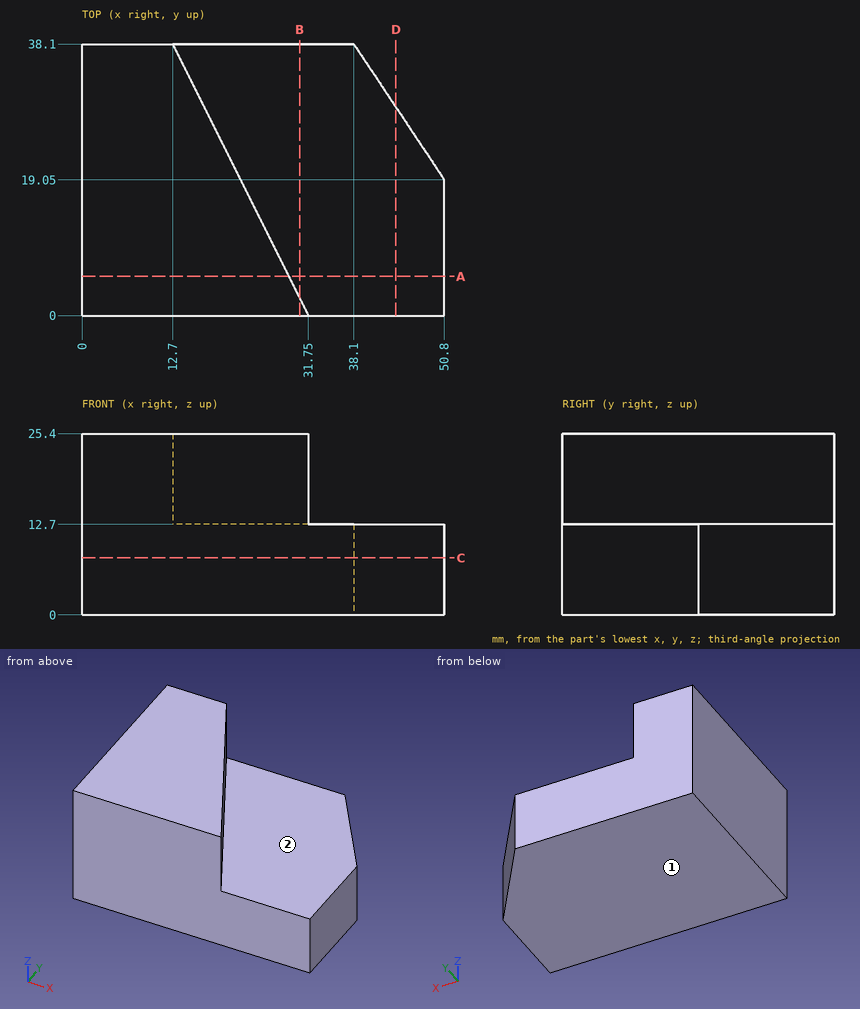
Input: dimensioned drawing with shaded views. Units: mm. Origin: part minimum x, y, z. A direction names the side the tool comes from. Round coordinates to 2 decimals unless told otherwise and drop trailing zeros. Order: outer loops, then holes, each group sorted by start corner. A loop starts at its lowest first (then second) coordinate and runs counter-clockwise, first axis right, second up. Notation, with made-up numbers: (-3, -34.75) - (48, -34.75) arc R4 cw to (48, -27.75) - close; hole circle Ø10 at (-32, -35). An arc over 180 degrees is marked (long way). Answer as a JSON object with one key per item and string values. Group by question number.
(1) Cut plane C-C (z = 8). Return loops of the section in (x, y).
(2) Cut plane B-B (x = 30.5). Return loops of the section in (y, z).
(3) Material intervals for probe 1 along Z at (x, y) = (30, 11); probe 2 along Y at (x, z) = (29.5, 16.25); probe 3 along X at (y, z) = (20, 20.5), sorted ascending. Write a range as from..to.
(4) Cut plane A-A (y = 5.5). Return loops of the section in (x, z).
(5) Pin query (flat end, axial travel): P1, Ø2, axis at x = 20.5, y = 28, coming from the +Z side; P2, Ø10, axis at y = 24.5, z = 13.5, coming from the +X side; P3, Ø12, axis at y = 32, z = 4.5, coming from the +X side. Return the tip coordinate at first contact, or that it passes through.
(6) Reachability of the marked faces 1 and 2 from +Z, -Z, +X, -X, +Y, -Y: full face, straight path, thin tool, end or side. Return the list, or none.
(7) Cut plane D-D (x = 44). Return loops of the section in (y, z), then the cut area to 3 significant figures.
Here are the results:
{
 "1": {"outline": "(0, 0) - (50.8, 0) - (50.8, 19.05) - (38.1, 38.1) - (0, 38.1) - close"},
 "2": {"outline": "(0, 0) - (38.1, 0) - (38.1, 12.7) - (2.5, 12.7) - (2.5, 25.4) - (0, 25.4) - close"},
 "3": {"probe 1": "z = 0..12.7", "probe 2": "y = 0..4.5", "probe 3": "x = 0..21.75"},
 "4": {"outline": "(0, 0) - (50.8, 0) - (50.8, 12.7) - (29, 12.7) - (29, 25.4) - (0, 25.4) - close"},
 "5": {"P1": "stops at z = 12.7", "P2": "stops at x = 50.46", "P3": "stops at x = 46.17"},
 "6": {"face 1": "-Z, +X, -X, +Y, -Y", "face 2": "+Z, +X, +Y"},
 "7": {"outline": "(0, 0) - (29.25, 0) - (29.25, 12.7) - (0, 12.7) - close", "area": "371 mm^2"}
}
